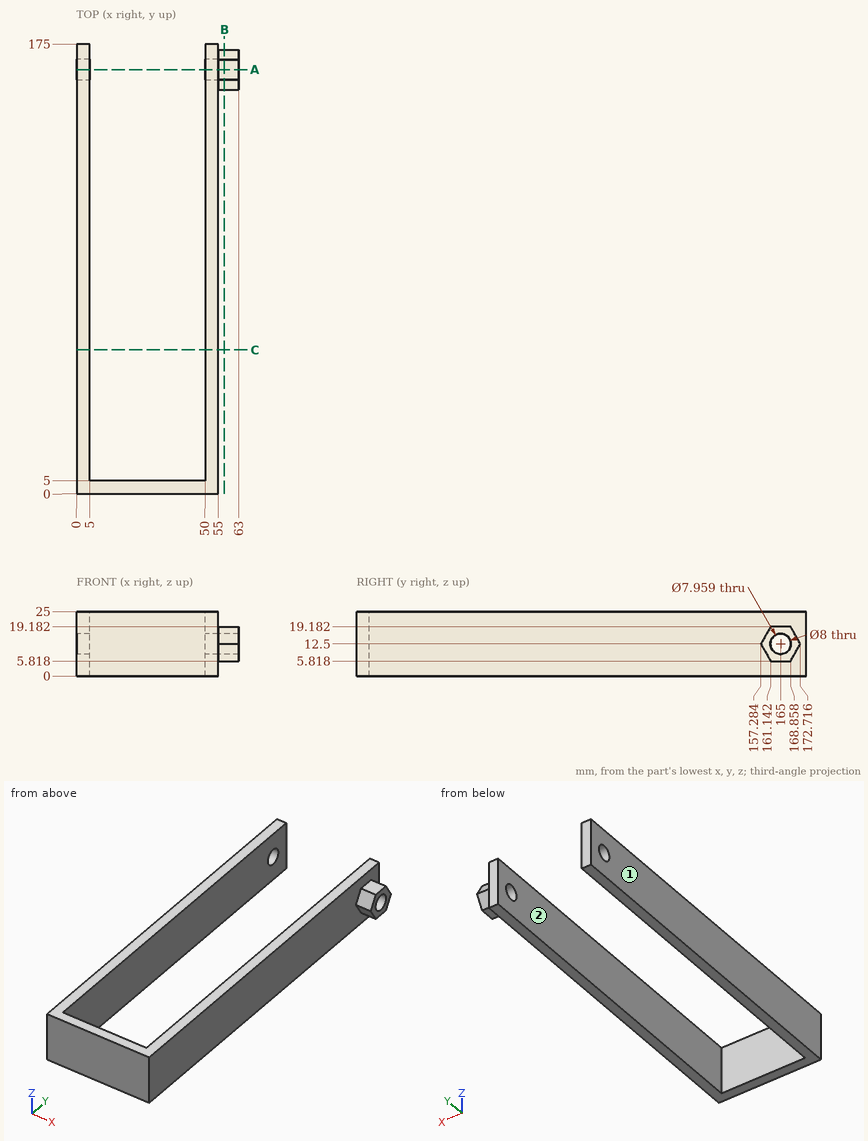
Geometry check sheet. Reference: drawing and pictorial views, mm from the part's lowest x, y, z. A direction names the side the tool comes from. Round coordinates to 2 decimals unless told otherwise and drop trailing zeros. Write each loop counter-clockwise with the first axis right and the second up, starting at its lowest first coordinate (ties: lowest second). Pieces come first, ordered by that corner, then holes.
(1) Access from +Z, -Z, +X, -X, +Y, -Y to the whole of each face (thin tool, end or side, straight path). Record for the marked faces 1 and 2.
Returned:
face 1: +Z, -Z, -X, +Y, -Y
face 2: +Z, -Z, +Y
(2) Material ranges on line 1 (X direction, y = 30, z = 17.5); line 2 (Z direction, x = 2, y = 165); line 3 (Y direction, x = 13.5, z = 16.5), recorded low to high.
Returned:
line 1: x = 0 to 5, 50 to 55
line 2: z = 0 to 8.5, 16.5 to 25
line 3: y = 0 to 5
(3) Section check C-C (y = 56). Enter the section's corners in (x, z), plus the area to 3 significant figures.
Returned:
outline: (0, 0) - (5, 0) - (5, 25) - (0, 25) - close; (50, 0) - (55, 0) - (55, 25) - (50, 25) - close
area: 250 mm2
(4) Section check A-A (y = 165). Give the number of separate pieces and of enclosed holes in the cut face, plus the area to 3 significant figures.
Returned:
separate pieces: 4
enclosed holes: 0
area: 213 mm2
(5) Section check B-B (x = 57.5). Enter the section's corners in (y, z) (1 decimal).
Returned:
outline: (157.3, 12.5) - (161.1, 5.8) - (168.9, 5.8) - (172.7, 12.5) - (168.9, 19.2) - (161.1, 19.2) - close; hole circle Ø8 at (165, 12.5)
(6) Depth check by flat-ended pin: pin 1 Ø4 at (x, z) = (20, 22) entering from +Y; pin 2 Ø7.5 at (y, z) = (54.5, 18) entering from +X; pin 3 Ø2.5 at (x, y) = (57, 163.5) entering from +Z. Enter the tip coordinate at first touch or a pass-through.
Returned:
pin 1: stops at y = 5
pin 2: stops at x = 55
pin 3: stops at z = 19.18
